```python
from build123d import *

# Parameters (mm, degrees)
ESQUISSE1_R                  = 2.5
BOSS_EXTRU_1_DEPTH           = 61
ESQUISSE2_W                  = 116
ESQUISSE2_H                  = 43
ENL_V_MAT_EXTRU_1_DEPTH      = 29
ENL_V_MAT_EXTRU_1_DEPTH_BACK = 29


with BuildPart() as part:
    # Esquisse1 → Boss.-Extru.1 (new body, symmetric)
    with BuildSketch(Plane.XY):
        with BuildLine():
            Line((-5.300956284, 42.810669399), (-28, 0))
            Line((-28, 0), (28, 0))
            Line((28, 0), (5.300956284, 42.810669399))
            ThreePointArc((5.300956284, 42.810669399), (0, 46), (-5.300956284, 42.810669399))
        make_face()
        with Locations((0, 40)):
            Circle(ESQUISSE1_R, mode=Mode.SUBTRACT)
    extrude(amount=BOSS_EXTRU_1_DEPTH, both=True)

    # Esquisse2 → Enlèv. mat.-Extru.1 (cut, two sides)
    with BuildSketch(Plane(origin=(0, 0, 0), x_dir=(0, 0, -1), z_dir=(1, 0, 0))) as enl_v_mat_extru_1_sk:
        with Locations((0, 24.5)):
            Rectangle(ESQUISSE2_W, ESQUISSE2_H)
    extrude(amount=ENL_V_MAT_EXTRU_1_DEPTH, mode=Mode.SUBTRACT)
    extrude(enl_v_mat_extru_1_sk.sketch, amount=-ENL_V_MAT_EXTRU_1_DEPTH_BACK, mode=Mode.SUBTRACT)


solid = part.part
```
CAD build for the part. Positions are in the model's coordinates, mm. A direction names the side the tool comes from. Round coordinates to 2 decimals unless told otherwise and drop trailing zeros. Loops run counter-clockwise (first coordinate to the right, second up) from the corner with the lowest first, then second, coordinate; pieces in that order, holes last. Notation, with made-up numbers: M 79.5,0 L 131.5,0 A24 cw 131.5,36 Z; hole C 39,-34 d1. An arc over 180 degrees is marked long. Use a Markdown table: item, result. Add a question column.
(1) Flat gauge pins, fed straight in: pin 1 (8 mm diameter, centred on x = 0, y = 40, fed in from +Z); pin 2 (16 mm diameter, centred on x = 3.5, z = 9.5, fed in from +Y). Where does each tip first touch, or does it go through?
(2) Cut at D-D (x = -23). Give the cut face in (y, z).
(3) Drill centre lines: line 1 (Y direction, x = 0, z = 59.2); line 2 (Z direction, x = -16, y = 16); line 3 (Y direction, x = 6, z = 38). Where is each one in solid material? Low to high.
(4) Cut at A-A (x = 0). Give the cut face in (y, z), and give its area (3 significant figures).
(5) Cut at C-C (y = 40). Give the cut face in (x, z), and give its area (3 significant figures).
(6) Pull direction Z, two halves, no side cores. Call faces 3 (the face through (0, 46, 60)), 4 (the face through (0, 3, 1)), 5 (the face through (0, 18, -61)): +Z half, -Z half, draft (parallel to the pull), parting line (faces both ways), or undercut.
(7) Which spindle directions (+Z, -Z, +X, -X, +Y, -Y) get a long thin tool onto all of the face, cutting with end or side? Do faces 1 (the face through (0, 19, -58)), 2 (the face through (0, 46, -59)). Say none if no direction does.
(8) Cut at B-B (y = 15.5). Give the cut face in (x, z).
Geometry says:
| question | item | result |
|---|---|---|
| 1 | pin 1 | stops at z = 61 |
| 1 | pin 2 | stops at y = 3 |
| 2 | outline | M 0,-61 L 9.43,-61 L 9.43,-58 L 3,-58 L 3,58 L 9.43,58 L 9.43,61 L 0,61 Z |
| 3 | line 1 | y = 0 to 37.5, 42.5 to 46 |
| 3 | line 2 | z = -61 to -58, 58 to 61 |
| 3 | line 3 | y = 0 to 3 |
| 4 | outline | M 0,-61 L 37.5,-61 L 37.5,-58 L 3,-58 L 3,58 L 37.5,58 L 37.5,61 L 0,61 Z; M 42.5,-61 L 46,-61 L 46,-58 L 42.5,-58 Z; M 42.5,58 L 46,58 L 46,61 L 42.5,61 Z |
| 4 | area | 594 mm² |
| 5 | outline | M -6.79,-61 L -2.5,-61 L -2.5,-58 L -6.79,-58 Z; M -6.79,58 L -2.5,58 L -2.5,61 L -6.79,61 Z; M 2.5,-61 L 6.79,-61 L 6.79,-58 L 2.5,-58 Z; M 2.5,58 L 6.79,58 L 6.79,61 L 2.5,61 Z |
| 5 | area | 51.5 mm² |
| 6 | face 3 | draft |
| 6 | face 4 | undercut |
| 6 | face 5 | -Z half |
| 7 | face 1 | +X, -X, +Y |
| 7 | face 2 | +Z, -Z, +Y |
| 8 | outline | M -19.78,-61 L 19.78,-61 L 19.78,-58 L -19.78,-58 Z; M -19.78,58 L 19.78,58 L 19.78,61 L -19.78,61 Z |
